```python
from build123d import *

# Parameters (mm, degrees)
F1_DEPTH = 12.7
F2_R     = 3.556
F3_DEPTH = 62.993


# Not quite as in the source:
# - ends of sketch curves that miss each other by under 0.0002 mm in the source are joined


with BuildPart() as f1:
    # F0 (on Right) → F1 (new body, symmetric)
    with BuildSketch(Plane.YZ):
        with BuildLine():
            Line((0.762, 33.02), (0.762, 17.6402746))
            ThreePointArc((0.762, 17.6402746), (0, -7.73684), (-0.7620002868, 17.6402793716))
            Line((-0.7620002868, 17.6402793716), (-0.762, 33.02))
            Line((-0.762, 33.02), (-21.59, 33.02))
            Line((-21.59, 33.02), (-22.86, 31.75))
            Line((-22.86, 31.75), (-22.86, -10.922))
            Line((-22.86, -10.922), (-41.275, -17.78))
            Line((-41.275, -17.78), (-41.275, -29.972))
            Line((-41.275, -29.972), (41.275, -29.972))
            Line((41.275, -29.972), (41.275, -21.0566))
            Line((41.275, -21.0566), (40.4876, -20.2692))
            Line((40.4876, -20.2692), (40.4876, -17.2175678))
            Line((40.4876, -17.2175678), (22.86, -10.922))
            Line((22.86, -10.922), (22.86, 31.75))
            Line((22.86, 31.75), (21.59, 33.02))
            Line((21.59, 33.02), (0.762, 33.02))
        make_face()
    extrude(amount=F1_DEPTH, both=True)

    # F2 (on face) → F3 (cut, through all)
    with BuildSketch(Plane(origin=(0, 0, -29.972), x_dir=(1, 0, 0), z_dir=(0, 0, -1))):
        with Locations((0, 31.75)):
            Circle(F2_R)
        with Locations((0, -31.75)):
            Circle(F2_R)
    extrude(amount=-F3_DEPTH, mode=Mode.SUBTRACT)


solid = f1.part
```
For this review, take the finished solid that the model builds, in its own axes (mm). A direction names the side the tool comes from. Give positions to 0.01 mm unless a question says otherwise; leave off trailing zeros. Write each loop counter-clockwise with the first axis right and the second up, starting at its lowest first coordinate (ties: lowest second). Pieces come first, ordered by that corner, then holes. Notation, with made-up numbers: M 66,3.25 L 99,3.25 A12 ccw 99,16.25 Z; hole C 42.5,-10.75 d9. An arc over 180 degrees is marked long. Answer as CSV lines item,"result".
1. Consider section D-D, the plane x = -1.25. Write out the cut boundary in (y, z) (3 decimals), then the cut area to 3 significant figures.
Findings:
outline,"M -41.275,-29.972 L -35.079,-29.972 L -35.079,-15.473 L -41.275,-17.78 Z; M -28.421,-29.972 L 28.421,-29.972 L 28.421,-12.908 L 22.86,-10.922 L 22.86,31.75 L 21.59,33.02 L 0.762,33.02 L 0.762,17.64 A12.7 cw long -0.762,17.64 L -0.762,33.02 L -21.59,33.02 L -22.86,31.75 L -22.86,-10.922 L -28.421,-12.993 Z; M 35.079,-29.972 L 41.275,-29.972 L 41.275,-21.057 L 40.488,-20.269 L 40.488,-17.218 L 35.079,-15.286 Z"
area,"2,710 mm2"
2. Consider section C-C, the plane y = -31.75. Write out the cut boundary in (x, z).
Findings:
outline,"M -12.7,-29.97 L -3.56,-29.97 L -3.56,-14.23 L -12.7,-14.23 Z; M 3.56,-29.97 L 12.7,-29.97 L 12.7,-14.23 L 3.56,-14.23 Z"
3. For pin 1 (20.5 mm diameter, centred on y = 0, z = 4.96, fed in from +X); pin 2 (1.5 mm diameter, centred on x = 0, z = 7, fed in from +Y); pin 3 (12.5 mm diameter, centred on x = 1.5, z = 14.5, fed in from -Y); pin 4 (2 mm diameter, centred on x = 9, y = 25, fed in from +Z), all flat-tipped, find the tip position at first contact; note any pin that passes through.
Findings:
pin 1,"passes through"
pin 2,"stops at y = 22.86"
pin 3,"stops at y = -22.86"
pin 4,"stops at z = -11.33"
4. Draft analysis for pull direction Y (two halves, no side actions). For faces 1 (the cylindrical face through (0.178, 0.548, -7.725)), 2 (the flat face through (0, 41.275, -26)), 3 (the flat face through (0, -22.86, 11)), 4 (the flat face through (0, 0.762, 25)), state which applies: +Y half, -Y half, draft (parallel to the pull), parting line (faces both ways), or undercut.
Findings:
face 1,"undercut"
face 2,"+Y half"
face 3,"-Y half"
face 4,"undercut"
5. Consider section A-A, the plane z = 23.5. Write out the cut boundary in (x, y).
Findings:
outline,"M -12.7,-22.86 L 12.7,-22.86 L 12.7,-0.76 L -12.7,-0.76 Z; M -12.7,0.76 L 12.7,0.76 L 12.7,22.86 L -12.7,22.86 Z"
6. Consider section B-B, the plane x = -10. Write out the cut boundary in (y, z) (3 decimals), then the cut area to 3 significant figures.
Findings:
outline,"M -41.275,-29.972 L 41.275,-29.972 L 41.275,-21.057 L 40.488,-20.269 L 40.488,-17.218 L 22.86,-10.922 L 22.86,31.75 L 21.59,33.02 L 0.762,33.02 L 0.762,17.64 A12.7 cw long -0.762,17.64 L -0.762,33.02 L -21.59,33.02 L -22.86,31.75 L -22.86,-10.922 L -41.275,-17.78 Z"
area,"2,920 mm2"
7. Wall thickness on line 1 (Y direction, x = 0, z = -20) (3 decimals); line 2 (Y direction, x = -9.75, z = 18); line 3 (Y direction, x = 1, z = -18) (1 decimal): over which ranges is each line inside the solid? List them lowest first.
Findings:
line 1,"y = -41.275 to -35.306, -28.194 to 28.194, 35.306 to 40.488"
line 2,"y = -22.86 to -0.76, 0.76 to 22.86"
line 3,"y = -41.3 to -35.2, -28.3 to 28.3, 35.2 to 40.5"
8. For faces 5 (the flat face through (0, -0.762, 25)), 6 (the flat face through (0, 40.488, -19)), 7 (the cylindrical face through (-0.77, -28.28, -21.56)), list the 3-axis set-ups (+Z, -Z, +X, -X, +Y, -Y) from which the entire face can be reached by the end or side of a thin tool; tool diameter is ignored.
Findings:
face 5,"+Z, +X, -X"
face 6,"+Z, +X, -X, +Y"
face 7,"+Z, -Z"
